Answer from the drawing. Dimensions are ordinates in mm from the lowest x, y and z of the part. Coordinates: 2 decimals unless noted, no trailing zeros. Write each loop counter-clockwise with the first axis right and the second up, starting at its lowest first coordinate (ties: lowest second). Pieces come first, ordered by that corner, then holes.
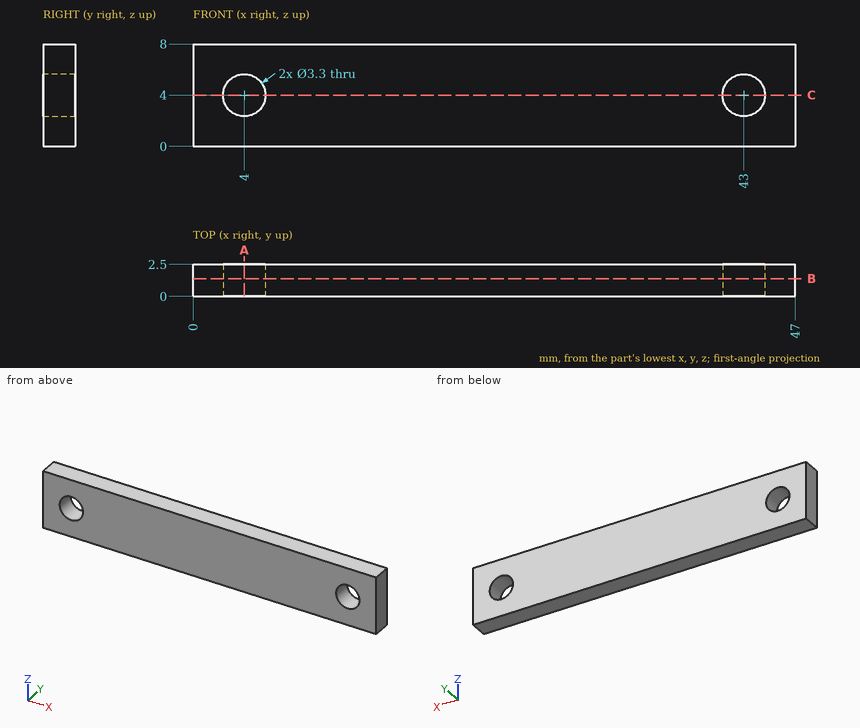
(1) Section B-B, the plane y = 1.4 is taken. Write down the section's boundary in (x, z), plus the area to 3 significant figures.
(2) Section A-A, the plane x = 4 is taken. Write down the section's boundary in (y, z), plus the area to 4 significant figures.
(3) Section C-C, the plane z = 4 is taken. Write down the section's boundary in (x, y).
(4) This flat-tipped pin is pushed along its axis until it touches: pin 1 (1 mm diameter, centred on x = 16.5, y = 1, fed in from -Z). Where does it stop, or does it pass through?
(5) Find the intervals of material crossed by probe 1 along X at (y, z) = (0.6, 4); probe 2 along Z at (x, y) = (4, 0.55); probe 3 along X at (y, z) = (1.6, 3.25), in increasing order.
Solution:
1. outline: (0, 0) - (47, 0) - (47, 8) - (0, 8) - close; hole circle Ø3.3 at (4, 4); hole circle Ø3.3 at (43, 4)
1. area: 359 mm2
2. outline: (0, 0) - (2.5, 0) - (2.5, 2.35) - (0, 2.35) - close; (0, 5.65) - (2.5, 5.65) - (2.5, 8) - (0, 8) - close
2. area: 11.75 mm2
3. outline: (0, 0) - (2.35, 0) - (2.35, 2.5) - (0, 2.5) - close; (5.65, 0) - (41.35, 0) - (41.35, 2.5) - (5.65, 2.5) - close; (44.65, 0) - (47, 0) - (47, 2.5) - (44.65, 2.5) - close
4. pin 1: stops at z = 0
5. probe 1: x = 0 to 2.35, 5.65 to 41.35, 44.65 to 47
5. probe 2: z = 0 to 2.35, 5.65 to 8
5. probe 3: x = 0 to 2.53, 5.47 to 41.53, 44.47 to 47
